```python
from build123d import *

# Parameters (mm, degrees)
SKETCH_1_R        = 40
EXTRUDE_1_DEPTH   = 20
FILLET_1_R        = 2
SWEEP_3_PROFILE_R = 0.75
SKETCH_2_W        = 0.5
SKETCH_2_H        = 1


with BuildPart() as part:
    # 草图1 → 凸台-拉伸1 (new body, symmetric)
    with BuildSketch(Plane(origin=(0, 0, 0), x_dir=(1, 0, 0), z_dir=(0, 1, 0))):
        Circle(SKETCH_1_R)
    extrude(amount=EXTRUDE_1_DEPTH, both=True)

    # 圆角1
    fillet_1_edges = [part.edges().sort_by_distance(p)[0] for p in [
        (-40, 20, 0),
    ]]
    fillet(fillet_1_edges, radius=FILLET_1_R)

    # 切除-扫描3: sweep along a path in 草图3
    with BuildLine(Plane.XZ.offset(20)) as sweep_3_path:
        CenterArc((0, 0), 9, 0, 360)
    # 切除-扫描3 profile (on start of the path) → 切除-扫描3 (sweep, cut)
    with BuildSketch(Plane(origin=(9, -20, 0), x_dir=(1, 0, 0), z_dir=(0, 0, 1))):
        Circle(SWEEP_3_PROFILE_R)
    sweep(path=sweep_3_path.line, mode=Mode.SUBTRACT)

    # 草图2 → 切除-旋转1 (revolve, cut)
    with BuildSketch(Plane.XY):
        with Locations((0.25, 0.5)):
            Rectangle(SKETCH_2_W, SKETCH_2_H)
    revolve(axis=Axis((0, 0, 0), (0, 1, 0)), mode=Mode.SUBTRACT)


solid = part.part
```
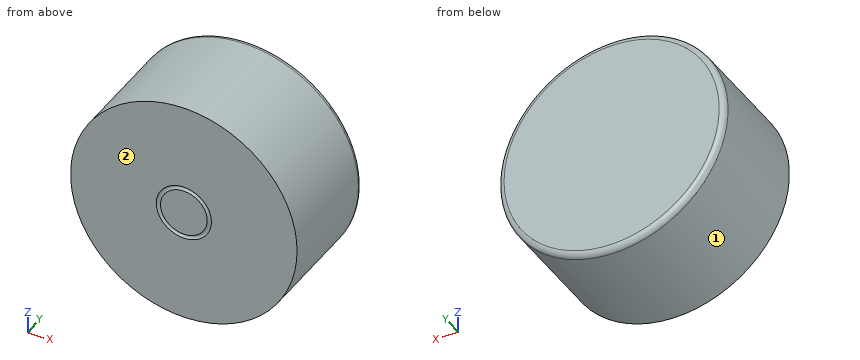
For this review, take the finished solid that the model builds, in its own axes (mm). Face numbers are marked on the shaded views. Coordinates: 2 decimals unless noted, no trailing zeros. Write each loop counter-clockwise with the first axis right and the second up, starting at its lowest first coordinate (ties: lowest second). Pieces come first, ordered by that corner, then holes.
(1) Wall thickness on probe 1 along Z at (x, y) = (0, 0.7); probe 2 along X at (y, z) = (-16, 17): over which ranges is each line inside the solid? List them lowest first.
(2) Add section A-A on y = -16.5. Give the boundary of the cut face in (x, z).
(3) The part is to be moulded in two halves that separate along Z. For the marked faces 1 and 2, say which applies: +Z half, -Z half, draft (parallel to the pull), parting line (faces both ways), or undercut.
(4) For pin 1 Ø1 at (y, z) = (14, -31.5) entering from +X; pin 2 Ø10 at (y, z) = (3, 15.5) entering from -X; pin 3 Ø4 at (y, z) = (-15.5, 19) entering from +X, all flat-tipped, find the tip position at first contact; note any pin that passes through.
Answer sheet:
1. probe 1: z = -40 to -0.5, 0.5 to 40
1. probe 2: x = -36.21 to 36.21
2. outline: circle Ø80 at (0, 0)
3. face 1: parting line
3. face 2: draft
4. pin 1: stops at x = 25.28
4. pin 2: stops at x = -38.6
4. pin 3: stops at x = 36.21
